Could you check a few things on this model? Use its own coordinates, in mm. Face numbers are marked on the shaded views. A direction names the side the tool comes from. Round coordinates to 2 decimals unless told otherwise and drop trailing zeros. Loops run counter-clockwise (first coordinate to the right, second up) from the corner with the lowest first, then second, coordinate; pieces in that order, holes last. Notation, with made-up numbers: (23.25, 77.25) -> (58.25, 77.25) arc R13 cw to (58.25, 87.25) -> close; hole circle Ø10 at (-1, -2). An arc over 180 degrees is marked (long way). One line per item, written item: value.
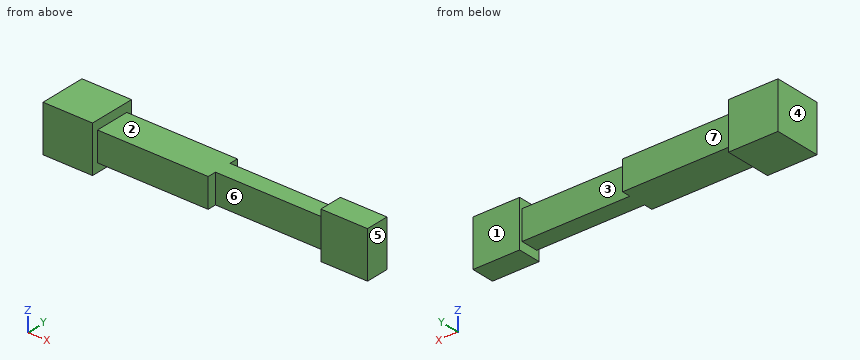
```python
from build123d import *

# Parameters (mm, degrees)
SKETCH1_W             = 17
SKETCH1_H             = 16
BOSS_EXTRUDE1_DEPTH   = 8
SKETCH1_W_2           = 16
SKETCH1_H_2           = 8
BOSS_EXTRUDE1_2_DEPTH = 8
SKETCH1_3_W           = 37
SKETCH1_3_H           = 6
BOSS_EXTRUDE2_DEPTH   = 5


with BuildPart() as part:
    # Sketch1 → Boss-Extrude1 (new, symmetric)
    with BuildSketch(Plane.XY):
        with Locations((-45.5, 0)):
            Rectangle(SKETCH1_W, SKETCH1_H)
    extrude(amount=BOSS_EXTRUDE1_DEPTH, both=True)



with BuildPart() as body_2:
    # Sketch1 → Boss-Extrude1 2 (new, symmetric)
    with BuildSketch(Plane.XY):
        with Locations((46, 0)):
            Rectangle(SKETCH1_W_2, SKETCH1_H_2)
    extrude(amount=BOSS_EXTRUDE1_2_DEPTH, both=True)


with BuildPart() as part_1:
    add(part.part)

    add(body_2.part)  # Boss-Extrude2 merges body 2
    # Sketch1<3> → Boss-Extrude2 (add, symmetric)
    with BuildSketch(Plane.XY):
        Polygon((1, -6), (1, -3), (1, 3), (1, 6), (-37, 6), (-37, -6), align=None)
        with Locations((19.5, 0)):
            Rectangle(SKETCH1_3_W, SKETCH1_3_H)
    extrude(amount=BOSS_EXTRUDE2_DEPTH, both=True)


solid = part_1.part
```
Item 1: For the marked faces 1, 2 and 3, which set-ups out of +Z, -Z, +X, -X, +Y, -Y let a thin tool reach every point of the face, with its end or its side?
Output:
face 1: +Z, -Z, +X, +Y
face 2: +Z, +Y, -Y
face 3: +Z, -Z, +Y
Item 2: I need wall thicknesses on line 1 (X direction, y = -3.5, z = -7.5); line 2 (X direction, y = -3.25, z = 0); line 3 (Y direction, x = 46, z = 1). Which ranges of each line are inside material? Lowest first, please. Write a range as from..to.
Output:
line 1: x = -54..-37, 38..54
line 2: x = -54..1, 38..54
line 3: y = -4..4
Item 3: If we section it at A-A on z = 2: List the corners of the cut face in (x, y) for me, plus the area to 3 significant figures.
Output:
outline: (-54, -8) -> (-37, -8) -> (-37, -6) -> (1, -6) -> (1, -3) -> (38, -3) -> (38, -4) -> (54, -4) -> (54, 4) -> (38, 4) -> (38, 3) -> (1, 3) -> (1, 6) -> (-37, 6) -> (-37, 8) -> (-54, 8) -> close
area: 1,080 mm²
Item 4: If we section it at C-C on x = 14.5: List the corners of the cut face in (y, z) for me.
Output:
outline: (-3, -5) -> (3, -5) -> (3, 5) -> (-3, 5) -> close
Item 5: If we section it at B-B on y = 0.5: List the corners of the cut face in (x, z) for me.
Output:
outline: (-54, -8) -> (-37, -8) -> (-37, -5) -> (38, -5) -> (38, -8) -> (54, -8) -> (54, 8) -> (38, 8) -> (38, 5) -> (-37, 5) -> (-37, 8) -> (-54, 8) -> close
Item 6: Will these pins go through, and if not, where does the flat tip stop? pin 1 Ø3 at (x, y) = (13.5, -2.5) entering from +Z; pin 2 Ø5 at (x, z) = (26, -0.5) entering from +Y; pin 3 Ø8 at (x, z) = (4.5, -1) entering from -Y.
Output:
pin 1: stops at z = 5
pin 2: stops at y = 3
pin 3: stops at y = -6
Item 7: If we mould it in two halves opening along X, with no side actions, what happens to the marked faces 4, 5, 6 and 7? For each: released by +X, released by -X, zero draft, split by the parting line, or undercut.
Output:
face 4: released by -X
face 5: released by +X
face 6: undercut
face 7: zero draft
